For this review, take the finished solid that the model builds, in its own axes (mm). Face numbers are marked on the shaded views. A direction names the side the tool comes from. Coordinates: 2 decimals unless noted, no trailing zeros. Loops run counter-clockwise (first coordinate to the right, second up) from the corner with the lowest first, then second, coordinate; pieces in that order, holes last. Notation, with made-up numbers: M -17.75,51 L 40.25,51 A27 cw 40.25,68 Z; hole C -32,85 d11. An arc over 180 degrees is marked long. Answer as a JSON object with one key per item and string values. Group by question number.
Item 1: Add section C-C (y = -5). State the section outline as (x, z) points, then the cut area to 3 significant figures.
Item 2: Insertion check: pin 1 (4 mm diameter, centred on x = -2.5, y = 1.5, fed in from +Z); pin 2 (7 mm diameter, centred on x = 1, y = -0.5, fed in from -Z); pin 3 (0.8 mm diameter, centred on y = 1.5, z = -14, fed in from -X); pin 4 (4 mm diameter, centred on x = 9, z = -37, fed in from -Y). Each pin has a flat end and moves straight along its axis. Give the tip position at first contact, or say it passes through.
Item 3: Tool access review of the marked faces 3 and 4: name each direction out of +Z, -Z, +X, -X, +Y, -Y from which nothing blocks a thin tool from reaching the whole face with its end or side.
Item 4: Add section A-A (x = 0). State the section outline as (y, z) points (3 decimals).
Item 5: Wall thickness on L1, parallel to Y at x = 0, z = -47 (3 decimals); L2, parallel to Z at x = 1.5, y = -4; L3, parallel to Y at x = 1.75, z = -22: over which ranges is each line inside the solid? List them lowest first. Write a range as from..to.
Item 6: Mouldability with a two-part tool opening along X and no side actions: class the marked faces 1 and 2 as +X half, -X half, draft (parallel to the pull), parting line (faces both ways), or undercut.
Item 7: Add section B-B (z = -4). State the section outline as (x, y) points, then the cut area to 3 significant figures.
Item 8: Add section D-D (x = -10.75). State the section outline as (y, z) points.
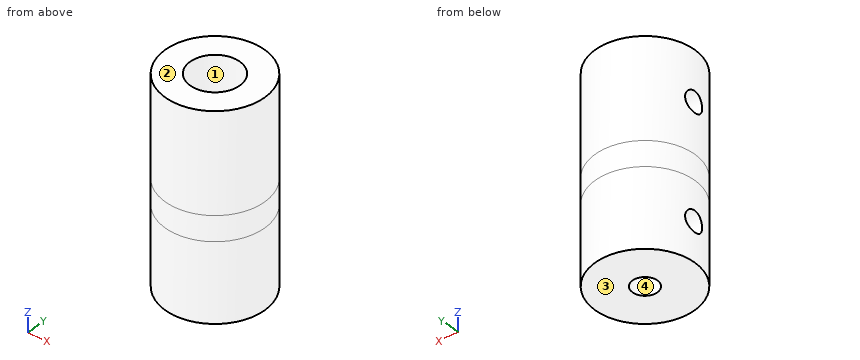
Autodesk Inventor part; units mm, degrees
ref_plane "XZ Plane" through (0, 0, 0) normal (0, 1, 0) x (-1, 0, 0)
ref_plane "XY Plane" through (0, 0, 0) normal (0, 0, 1) x (1, 0, 0)
sketch "Sketch1" plane through (0, 0, 0) normal (0, 0, 1) x (1, 0, 0)
  circle A0 centre (0, 0) radius 12.7
  circle A1 centre (0, 0) radius 6.35
  dimension "d0" = 25.4
  dimension "d1" = 12.7
extrude "Extrusion1" add sketch "Sketch1" against normal blind 25.4
sketch "Sketch2" plane through (0, 0, 0) normal (0, 1, 0) x (-1, 0, 0)
  point P0 (0, 0)
ref_plane "Work Plane2" through (-12.7, 0, 0) normal (1, 0, 0) x (0, 1, 0)
ref_plane "Work Plane1" through (-6.35, 0, 0) normal (1, 0, 0) x (0, 1, 0)
sketch "Sketch3" plane through (-6.35, 0, 0) normal (1, 0, 0) x (0, 1, 0)
  line L0 (-12.7, -25.4) -> (12.7, -25.4) construction
  line L1 (0, -25.4) -> (0, 0) construction
  circle A0 centre (0, -12.7) radius 2.55
  dimension "d6" = 5.1
sketch "Sketch4" plane through (-12.7, 0, 0) normal (1, 0, 0) x (0, 1, 0)
  line L0 (-12.7, -25.4) -> (12.7, -25.4) construction
  line L1 (0, -25.4) -> (0, 0) construction
  circle A0 centre (0, -12.7) radius 2.65
  dimension "d7" = 5.3
loft "Loft1" cut profiles "Sketch3", "Sketch4"
sketch "Sketch5" plane through (0, 0, -25.4) normal (0, 0, -1) x (-1, 0, 0)
  circle A0 centre (0, 0) radius 6.35
  circle A1 centre (0, 0) radius 12.7
extrude "Extrusion2" add sketch "Sketch5" along normal blind 6.35 contours A0 | A1
sketch "Sketch6" plane through (0, 0, -31.75) normal (0, 0, -1) x (-1, 0, 0)
  circle A0 centre (0, 0) radius 12.7
  circle A1 centre (0, 0) radius 3.175
  dimension "d14" = 6.35
extrude "Extrusion3" add sketch "Sketch6" along normal blind 20
sketch "Sketch7" plane through (-6.35, 0, 0) normal (1, 0, 0) x (0, 1, 0)
  line L0 (-12.7, -51.75) -> (12.7, -51.75) construction
  line L1 (0, -51.75) -> (0, -31.75) construction
  line L2 (-3.175, -31.75) -> (3.175, -31.75) construction
  circle A0 centre (0, -41.75) radius 2.55
  point P0 (0, 0)
  dimension "d17" = 5.1
sketch "Sketch8" plane through (-12.7, 0, 0) normal (1, 0, 0) x (0, 1, 0)
  line L0 (-12.7, -51.75) -> (12.7, -51.75) construction
  line L1 (0, -51.75) -> (0, -31.75) construction
  line L2 (-3.175, -31.75) -> (3.175, -31.75) construction
  circle A0 centre (0, -41.75) radius 2.65
  point P0 (0, 0)
  dimension "d18" = 5.3
loft "Loft2" cut profiles "Sketch7", "Sketch8"
properties part number "Threaded Rod Coupler"
From the geometry:
{
 "1": {"outline": "M -11.67,-51.75 L 11.67,-51.75 L 11.67,0 L 3.91,0 L 3.91,-25.4 L -3.91,-25.4 L -3.91,0 L -11.67,0 Z", "area": "1,010 mm²"},
 "2": {"pin 1": "stops at z = -25.4", "pin 2": "stops at z = -51.75", "pin 3": "stops at x = -6.35", "pin 4": "stops at y = -10.6"},
 "3": {"face 3": "-Z, +X, -X, +Y, -Y", "face 4": "-Z"},
 "4": {"outline": "M -12.7,-51.75 L -3.175,-51.75 L -3.175,-31.75 L 3.175,-31.75 L 3.175,-51.75 L 12.7,-51.75 L 12.7,0 L 6.35,0 L 6.35,-25.4 L -6.35,-25.4 L -6.35,0 L -12.7,0 Z"},
 "5": {"L1": "y = -12.7..-3.175, 3.175..12.7", "L2": "z = -51.75..-25.4", "L3": "y = -12.58..-6.1, 6.1..12.58"},
 "6": {"face 1": "undercut", "face 2": "draft"},
 "7": {"outline": "C 0,0 d25.4; hole C 0,0 d12.7", "area": "380 mm²"},
 "8": {"outline": "M -6.76,-51.75 L 6.76,-51.75 L 6.76,0 L -6.76,0 Z; hole C 0,-41.75 d5.24; hole C 0,-12.7 d5.24"}
}
